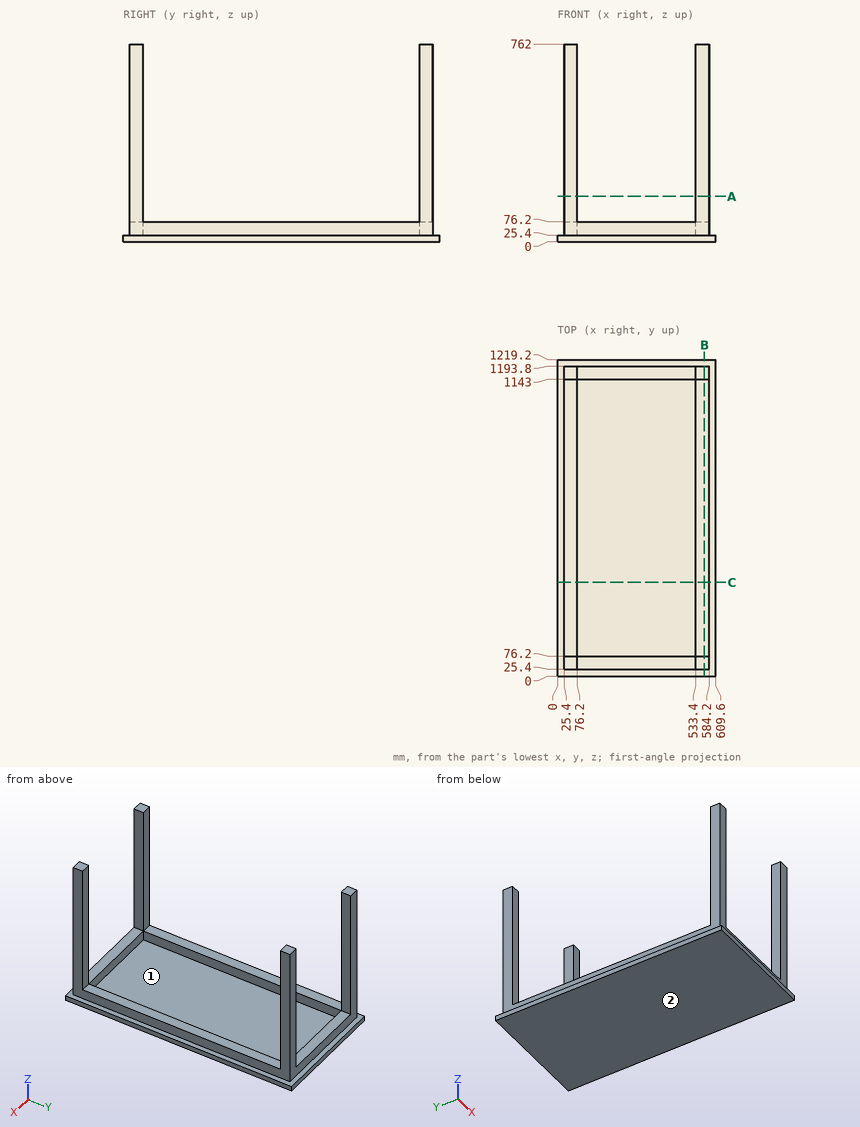
Geometry check sheet. Reference: drawing and pictorial views, mm from the part's lowest x, y, z. Coordinates: 2 decimals unless noted, no trailing zeros. Order: outer loops, then holes, each group sorted by start corner. A loop starts at its lowest first (then second) coordinate and runs counter-clockwise, first axis right, second up. Notation, with made-up numbers: (62, 38) - (115, 38) arc R14 ccw to (115, 57) - close; hole circle Ø4 at (53, 62.25). An arc over 180 degrees is marked (long way). Answer in a Markdown table with one row per item. Add a question column.
1) Gauge pin test, flat ends, axial feed: P1, Ø15, axis at x = 300.5, z = 42, coming from the +Y side; P2, Ø3, axis at x = 254, y = 766.5, coming from the +Z side. Record the tip position at first contact, or that the pin passes through.
2) Release check for a two-part mould opening along Y. For the marked faces 1 and 2 record: +Y half, -Y half, draft (parallel to the pull), parting line (faces both ways), or undercut.
3) Cross-section at A-A, the plane z = 175. Record the cut outline in (x, y), then the cut area to 3 significant figures.
4) Cross-section at B-B, the plane x = 565.5. Record the cut outline in (y, z).
5) Material ranges on line 1 along Y through (x, z) = (571.5, 155); line 2 along Z through (x, y) = (420, 1060); line 3 along X through (y, z) = (636, 39.5), recorded low to high. Write a range as [from, to].
6) Cross-section at C-C, the plane y = 361. Record the cut outline in (x, z).
Check result:
| question | item | result |
|---|---|---|
| 1 | P1 | stops at y = 1193.8 |
| 1 | P2 | stops at z = 25.4 |
| 2 | face 1 | undercut |
| 2 | face 2 | draft |
| 3 | outline | (25.4, 25.4) - (76.2, 25.4) - (76.2, 76.2) - (25.4, 76.2) - close; (25.4, 1143) - (76.2, 1143) - (76.2, 1193.8) - (25.4, 1193.8) - close; (533.4, 25.4) - (584.2, 25.4) - (584.2, 76.2) - (533.4, 76.2) - close; (533.4, 1143) - (584.2, 1143) - (584.2, 1193.8) - (533.4, 1193.8) - close |
| 3 | area | 10,300 mm² |
| 4 | outline | (0, 0) - (1219.2, 0) - (1219.2, 25.4) - (1193.8, 25.4) - (1193.8, 762) - (1143, 762) - (1143, 76.2) - (76.2, 76.2) - (76.2, 762) - (25.4, 762) - (25.4, 25.4) - (0, 25.4) - close |
| 5 | line 1 | y = [25.4, 76.2], [1143, 1193.8] |
| 5 | line 2 | z = [0, 25.4] |
| 5 | line 3 | x = [25.4, 76.2], [533.4, 584.2] |
| 6 | outline | (0, 0) - (609.6, 0) - (609.6, 25.4) - (584.2, 25.4) - (584.2, 76.2) - (533.4, 76.2) - (533.4, 25.4) - (76.2, 25.4) - (76.2, 76.2) - (25.4, 76.2) - (25.4, 25.4) - (0, 25.4) - close |
